Geometry: final body of the model. Coordinates: model frame, mm. Give positions to 0.01 mm unless a question says otherwise; leave off trailing zeros. Write each loop counter-clockwise with the first axis right and the second up, starting at its lowest first coordinate (ties: lowest second). Pieces come first, ordered by that corner, then holes. Notation, with made-up numbers: (80, 71.5) -> (127, 71.5) arc R24 cw to (127, 106.5) -> close; hole circle Ø6 at (-36, 79.5). An arc over 180 degrees is marked (long way). Answer as a JSON object with one key per item and string values. Group by question number.
(1) Section query C-C on x = -12. Output: boundary loops of the cut face in (y, z), plus the area to 3 significant figures.
(2) Material intervals for probe 1 along X at (y, z) = (4, -15); probe 2 along X at (y, z) = (2.5, -13); probe 3 along Z at (x, y) = (-17, 8), sorted ascending.
(3) Section query A-A on y = 2. Output: boundary loops of the cut face in (x, z), plus the area to 3 significant figures.
(4) Section query B-B on z = -9.5. Output: boundary loops of the cut face in (x, y), plus the area to 3 significant figures.
from build123d import *

# Parameters (mm, degrees)
SKETCH6_W           = 42.426406872
SKETCH6_H           = 42.426406872
BOSS_EXTRUDE4_DEPTH = 30
CUT_EXTRUDE2_DEPTH  = 43.426406871


with BuildPart() as part:
    # Sketch6 → Boss-Extrude4 (new body)
    with BuildSketch(Plane(origin=(0, 0, 0), x_dir=(1, 0, 0), z_dir=(0, 1, 0))):
        Rectangle(SKETCH6_W, SKETCH6_H)
    extrude(amount=BOSS_EXTRUDE4_DEPTH)

    # Sketch7 → Cut-Extrude2 (cut, through all)
    with BuildSketch(Plane.XZ):
        Polygon((-21.213203436, -8.786796564), (-8.786796564, -21.213203436), (-21.213203436, -21.213203436), align=None)
    extrude(amount=-CUT_EXTRUDE2_DEPTH, mode=Mode.SUBTRACT)


solid = part.part
Answer list:
{
 "1": {"outline": "(0, -18) -> (30, -18) -> (30, 21.21) -> (0, 21.21) -> close", "area": "1,180 mm2"},
 "2": {"probe 1": "-15 to 21.21", "probe 2": "-17 to 21.21", "probe 3": "-13 to 21.21"},
 "3": {"outline": "(-21.21, -8.79) -> (-8.79, -21.21) -> (21.21, -21.21) -> (21.21, 21.21) -> (-21.21, 21.21) -> close", "area": "1,720 mm2"},
 "4": {"outline": "(-20.5, 0) -> (21.21, 0) -> (21.21, 30) -> (-20.5, 30) -> close", "area": "1,250 mm2"}
}
